from build123d import *

# Parameters (mm, degrees)
BOSS_EXTRUDE1_DEPTH   = 50
M3X0_5_TAPPED_HOLE1_D = 2.5


with BuildPart() as part:
    # Sketch1 → Boss-Extrude1 (new body)
    with BuildSketch(Plane.XY):
        Polygon((3.175426481, 0), (1.58771324, 2.75), (-1.58771324, 2.75), (-3.175426481, 0), (-1.58771324, -2.75), (1.58771324, -2.75), align=None)
    extrude(amount=BOSS_EXTRUDE1_DEPTH)

    # M3x0.5 Tapped Hole1 (through all)
    with Locations(Plane.XY.offset(50)):
        with Locations((0, 0)):
            Hole(M3X0_5_TAPPED_HOLE1_D / 2)


solid = part.part
Geometry check sheet. Reference: the model listing, model coordinates, mm. Round coordinates to 2 decimals unless told otherwise and drop trailing zeros. Order: outer loops, then holes, each group sorted by start corner. A loop starts at its lowest first (then second) coordinate and runs counter-clockwise, first axis right, second up. Notation, with made-up numbers: M 43,33 L 89,33 A12 cw 89,55 Z; hole C 61,57 d9. An arc over 180 degrees is marked long. Write each question's results on one line, items separated by ' | '. Start each with the question number.
1. Cross-section at C-C on x = -2. Record the boundary of the cut face in (y, z), plus the area to 3 significant figures.
2. Material ranges on L1, parallel to Y at x = 0, z = 14.5; L2, parallel to X at y = -0.3, z = 20; L3, parallel to X at y = -1.1, z = 8.5, recorded low to high. Write a range as from..to.
3. Go/stop test with a flat-tipped pin: P1, Ø1.5, axis at y = 1.5, z = 7, coming from the +X side. Record where the tip stops, or that it passes through.
4. Cross-section at A-A on x = 0. Record the boundary of the cut face in (y, z).
5. Cross-section at B-B on z = 6. Record the boundary of the cut face in (x, y).
6. Draft check along Y on faces 1 (the face through (-2.37, 1.394, 24.65)), 2 (the face through (0.27, -1.22, 24.65)), 3 (the face through (1, 1, 50)). Enter one of: pulls with the +Y half, pulls with the -Y half, needs draft (parallel to the pull), parting line crosses it, or undercut.
7. Cross-section at D-D on y = 2.2. Record the boundary of the cut face in (x, z).
Resolved:
1) outline: M -2.04,0 L 2.04,0 L 2.04,50 L -2.04,50 Z | area: 204 mm2
2) L1: -2.75..-1.25, 1.25..2.75 | L2: -3..-1.21, 1.21..3 | L3: -2.54..-0.59, 0.59..2.54
3) P1: x = 2.74
4) outline: M -2.75,0 L -1.25,0 L -1.25,50 L -2.75,50 Z; M 1.25,0 L 2.75,0 L 2.75,50 L 1.25,50 Z
5) outline: M -3.18,0 L -1.59,-2.75 L 1.59,-2.75 L 3.18,0 L 1.59,2.75 L -1.59,2.75 Z; hole C 0,0 d2.5
6) face 1: pulls with the +Y half | face 2: undercut | face 3: needs draft
7) outline: M -1.91,0 L 1.91,0 L 1.91,50 L -1.91,50 Z
